Part model, mm, in its own coordinate system. A direction names the side the tool comes from. Round coordinates to 2 decimals unless told otherwise and drop trailing zeros. Order: outer loops, then holes, each group sorted by start corner. A loop starts at its lowest first (then second) coordinate and runs counter-clockwise, first axis right, second up. Notation, with made-up numbers: (5.5, -30) - (52.5, -30) arc R14 ccw to (52.5, -3) - close; hole circle Ø11 at (-4.75, 3.5). An arc over 180 degrees is marked (long way). Answer as a JSON object with one key per item and string values.
```python
from build123d import *

# Parameters (mm, degrees)
F0_W     = 79
F0_H     = 59
F0_W_2   = 75
F0_H_2   = 55
F1_DEPTH = 4
F0_W_3   = 83
F0_H_3   = 63
F2_DEPTH = 2


with BuildPart() as f1:
    # F0 (on Top) → F1 (new body)
    with BuildSketch(Plane.XY):
        with Locations((1.25, 1)):
            Rectangle(F0_W, F0_H)
        with Locations((1.25, 1)):
            Rectangle(F0_W_2, F0_H_2, mode=Mode.SUBTRACT)
        with Locations((1.25, 1)):
            Rectangle(F0_W_2, F0_H_2)
    extrude(amount=F1_DEPTH)

    # F0 (on Top) → F2 (join)
    with BuildSketch(Plane.XY):
        with Locations((1.25, 1)):
            Rectangle(F0_W_3, F0_H_3)
        with Locations((1.25, 1)):
            Rectangle(F0_W, F0_H, mode=Mode.SUBTRACT)
    extrude(amount=F2_DEPTH)


solid = f1.part
```
Item 1: Cut at B-B (y = -9.5). Write the cut outline in (x, z).
Taken from the geometry:
{"outline": "(-40.25, 0) - (42.75, 0) - (42.75, 2) - (40.75, 2) - (40.75, 4) - (-38.25, 4) - (-38.25, 2) - (-40.25, 2) - close"}
Item 2: Probe L1, parallel to Y at x = -15, z = 3.45; L2, parallel to X at y = 14, z = 2.15. List the from-to ranges inside material, lowest first. Write a range as from..to.
Taken from the geometry:
{"L1": "-28.5..30.5", "L2": "-38.25..40.75"}
Item 3: Cut at C-C (z = 3.2). Write the cut outline in (x, y), plus the area to 3 significant figures.
Taken from the geometry:
{"outline": "(-38.25, -28.5) - (40.75, -28.5) - (40.75, 30.5) - (-38.25, 30.5) - close", "area": "4,660 mm2"}
Item 4: Cut at A-A (x = -19). Write the cut outline in (y, z), plus the area to 3 significant figures.
Taken from the geometry:
{"outline": "(-30.5, 0) - (32.5, 0) - (32.5, 2) - (30.5, 2) - (30.5, 4) - (-28.5, 4) - (-28.5, 2) - (-30.5, 2) - close", "area": "244 mm2"}
Item 5: Tool access for faces 1 (the flat face through (1, 30.5, 3)), 2 (the flat face through (1, -28.5, 3)), 3 (the flat face through (-38.25, 1, 3)), 4 (the flat face through (1, 32.5, 1)), 5 (the flat face through (40.75, 1, 3)): list every direction of +Z, -Z, +X, -X, +Y, -Y with a clear straight run to the whole face (end or side of a thin tool).
Taken from the geometry:
{"face 1": "+Z, +X, -X, +Y", "face 2": "+Z, +X, -X, -Y", "face 3": "+Z, -X, +Y, -Y", "face 4": "+Z, -Z, +X, -X, +Y", "face 5": "+Z, +X, +Y, -Y"}
Item 6: Drop flat-ended pins along their axis: P1, Ø0.6, axis at y = 8, z = 3.5, coming from the -X side; P2, Ø0.6, axis at x = 7, z = 3, coming from the -Y side; P3, Ø1.6, axis at x = 12, z = 3, coming from the +Y side. Give the stop position or say it passes through.
Taken from the geometry:
{"P1": "x = -38.25", "P2": "y = -28.5", "P3": "y = 30.5"}
